```python
from build123d import *

# Parameters (mm, degrees)
BOX006_W             = 25
BOX006_H             = 10
BOX006_DEPTH         = 10
CHAMFER003_SIZE      = 7
FILLET002003_R       = 8
FILLET002008005008_R = 1


with BuildPart() as part:
    # Box006 → Box006 (new body)
    with BuildSketch(Plane(origin=(85, 5, 30), x_dir=(1, 0, 0), z_dir=(0, 0, 1))):
        with Locations((12.5, 5)):
            Rectangle(BOX006_W, BOX006_H)
    extrude(amount=BOX006_DEPTH)

    # Chamfer003
    chamfer003_edges = [part.edges().sort_by_distance(p)[0] for p in [
        (85, 10, 40),
        (110, 10, 40),
    ]]
    chamfer(chamfer003_edges, length=CHAMFER003_SIZE)

    # Fillet002003
    fillet002003_edges = [part.edges().sort_by_distance(p)[0] for p in [
        (92, 10, 40),
        (103, 10, 40),
    ]]
    fillet(fillet002003_edges, radius=FILLET002003_R)


with BuildPart() as part_1:
    # Fillet002003 placement: moved
    add(part.part.moved(Location((-7.5, 0, -3))))

    # Fillet002008005008
    fillet002008005008_edges = [part_1.edges().sort_by_distance(p)[0] for p in [
        (95.247759, 5, 36.391036),
        (95.247759, 15, 36.391036),
    ]]
    fillet(fillet002008005008_edges, radius=FILLET002008005008_R)


with BuildPart() as part_2:
    # Fillet002008005008 placement: moved
    add(part_1.part.moved(Location((5, 0, -22.5))))


solid = part_2.part
```
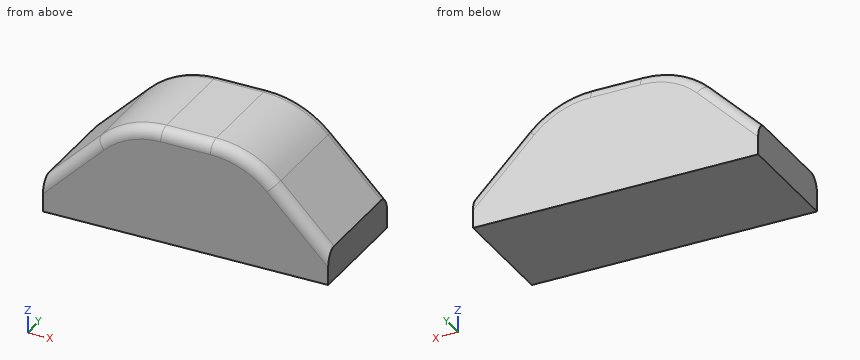
Can you work these out from the model? Positions are in its coordinate system, mm. Give positions to 0.01 mm unless a question says otherwise; leave off trailing zeros. Order: outer loops, then holes, each group sorted by start corner. A loop starts at its lowest first (then second) coordinate and runs counter-clockwise, first axis right, second up. Notation, with made-up numbers: M -36.5,15.25 L -31.5,15.25 A23 ccw -31.5,49.25 Z; hole C 50,79.5 d2. An arc over 180 degrees is marked long. Write item = value, one per line. Start each with the question number.
Q1. I need wall thicknesses on probe 1 along Z at (x, y) = (89.25, 10.75); probe 2 along X at (y, z) = (14.25, 9.25); probe 3 along X at (y, z) = (13.5, 11.75). Which ranges of each line are inside material? Lowest first, please. Write a range as [from, to].
Q2. Will this pin go through, and if not, where does the flat tip stop? pin 1 Ø1 at (y, z) = (11.5, 13.5) entering from +X.
Q3. Suppose I cut it at A-A (y = 10.75). Write out the boundary of the cut face in (x, z).
Check result:
q1.probe_1 = [4.5, 13.66]
q1.probe_2 = [84.29, 105.71]
q1.probe_3 = [86.75, 103.25]
q2.pin_1 = 101.85
q3.outline = M 82.5,4.5 L 107.5,4.5 L 107.5,7.5 L 102.84,12.16 A8 ccw 97.19,14.5 L 92.81,14.5 A8 ccw 87.16,12.16 L 82.5,7.5 Z
